Part model, mm, in its own coordinate system. A direction names the side the tool comes from. Round coordinates to 2 decimals unless told otherwise and drop trailing zeros. Write each loop counter-clockwise with the first axis right and the second up, starting at its lowest first coordinate (ties: lowest second). Pieces come first, ordered by that corner, then holes.
1) Flat gauge pins, fed straight in: pin 1 (3 mm diameter, centred on x = 5.5, z = -0.5, fed in from +Y); pin 2 (3.5 mm diameter, centred on x = 24.97, y = 15, fed in from -Z); pin 3 (1.5 mm diameter, centred on y = 10, z = -1.5, fed in from +X). Where does each tip first touch, or does it go through?
2) Saw through at C-C on y = 7.5. Write the cut outline in (x, z).
3) Saw through at D-D on y = 5. Write the cut outline in (x, z), and give its area (3 significant figures).
4) Saw through at A-A on y = 15. Write the cut outline in (x, z), and give its area (3 significant figures).
5) Which spindle directions (+Z, -Z, +X, -X, +Y, -Y) get a long thin tool onto all of the face, cutting with end or side? Do faces 4 (the flat face through (24, 10, 0)), 5 (the flat face through (10.4, 9, -2.2)), 6 (the flat face through (16.77, 4, 0)). Say none if no direction does.
6) Pull direction Z, two halves, no side cores. Call faces 1 (the flat face through (1.17, 10, -3)), 2 (the flat face through (11, 15, -2.5)), 3 (the flat face through (-3, 10, 0)): +Z half, -Z half, draft (parallel to the pull), parting line (faces both ways), or undercut.
7) Drill centre lines: L1, parallel to X at y = 8.25, z = -1.5; L2, parallel to X at y = 16, z = -0.75; L3, parallel to Y at x = 25.5, z = 0.75. Where is each one in solid material? Low to high.
8) Saw through at B-B on z = -0.75. Write the cut outline in (x, y), and give its area (3 significant figures).
```python
from build123d import *

# Parameters (mm, degrees)
BOSS_EXTRUDE1_DEPTH = 20
SKETCH2_R           = 1.5
CUT_EXTRUDE1_DEPTH  = 16
CUT_EXTRUDE2_DEPTH  = 11


with BuildPart() as part:
    # Sketch1 → Boss-Extrude1 (new body)
    with BuildSketch(Plane(origin=(0, 0, 0), x_dir=(1, 0, 0), z_dir=(0, 1, 0))):
        Polygon((16.770422535, -3), (28.470422535, -3), (28.470422535, 0), (19.770422535, 0), (19.770422535, 5), (1.170422535, 5), (1.170422535, 0), (-7.529577465, 0), (-7.529577465, -3), (4.170422535, -3), (4.170422535, 2), (16.770422535, 2), align=None)
    extrude(amount=BOSS_EXTRUDE1_DEPTH)

    # Sketch2 → Cut-Extrude1 (cut)
    with BuildSketch(Plane(origin=(0, 0, 0), x_dir=(-1, 0, 0), z_dir=(0, 0, -1))):
        with Locations((4.029577465, 15)):
            Circle(SKETCH2_R)
        with Locations((4.029577465, 5)):
            Circle(SKETCH2_R)
        with Locations((-24.970422535, 5)):
            Circle(SKETCH2_R)
        with Locations((-24.970422535, 15)):
            Circle(SKETCH2_R)
    extrude(amount=-CUT_EXTRUDE1_DEPTH, mode=Mode.SUBTRACT)

    # Sketch3 → Cut-Extrude2 (cut)
    with BuildSketch(Plane(origin=(0, 20, 0), x_dir=(1, 0, 0), z_dir=(0, 1, 0))):
        Polygon((4.170422535, -3), (4.170422535, 2), (16.770422535, 2), (16.770422535, -3), (17.220422535, -3), (17.220422535, 2.5), (3.670422535, 2.5), (3.670422535, -3), align=None)
    extrude(amount=-CUT_EXTRUDE2_DEPTH, mode=Mode.SUBTRACT)


solid = part.part
```
Completed:
1. pin 1: stops at y = 9
1. pin 2: stops at z = 0
1. pin 3: stops at x = 19.77
2. outline: (-7.53, 0) - (1.17, 0) - (1.17, -5) - (19.77, -5) - (19.77, 0) - (28.47, 0) - (28.47, 3) - (16.77, 3) - (16.77, -2) - (4.17, -2) - (4.17, 3) - (-7.53, 3) - close
3. outline: (-7.53, 0) - (-5.53, 0) - (-5.53, 3) - (-7.53, 3) - close; (-2.53, 0) - (1.17, 0) - (1.17, -5) - (19.77, -5) - (19.77, 0) - (23.47, 0) - (23.47, 3) - (16.77, 3) - (16.77, -2) - (4.17, -2) - (4.17, 3) - (-2.53, 3) - close; (26.47, 0) - (28.47, 0) - (28.47, 3) - (26.47, 3) - close
3. area: 120 mm2
4. outline: (-7.53, 0) - (-5.53, 0) - (-5.53, 3) - (-7.53, 3) - close; (-2.53, 0) - (1.17, 0) - (1.17, -5) - (19.77, -5) - (19.77, 0) - (23.47, 0) - (23.47, 3) - (17.22, 3) - (17.22, -2.5) - (3.67, -2.5) - (3.67, 3) - (-2.53, 3) - close; (26.47, 0) - (28.47, 0) - (28.47, 3) - (26.47, 3) - close
4. area: 108 mm2
5. face 4: -Z, +X, +Y, -Y
5. face 5: +Z, +Y
5. face 6: +Z, +Y, -Y
6. face 1: draft
6. face 2: +Z half
6. face 3: -Z half
7. L1: x = 1.17 to 4.17, 16.77 to 19.77
7. L2: x = 1.17 to 3.67, 17.22 to 19.77
7. L3: y = 0 to 3.6, 6.4 to 13.6, 16.4 to 20
8. outline: (1.17, 0) - (4.17, 0) - (4.17, 9) - (3.67, 9) - (3.67, 20) - (1.17, 20) - close; (16.77, 0) - (19.77, 0) - (19.77, 20) - (17.22, 20) - (17.22, 9) - (16.77, 9) - close
8. area: 110 mm2
